Read the model definition and answer for the solid it produces. Units are mm, in the model's axes. A direction names the side the tool comes from. Coordinates: 2 decimals unless noted, no trailing zeros. Use CSV: the item, a comma, the result in double quotes.
Autodesk Inventor part; units mm, degrees
ref_plane "YZ Plane" through (0, 0, 0) normal (1, 0, 0) x (0, 1, 0)
ref_plane "XZ Plane" through (0, 0, 0) normal (0, 1, 0) x (-1, 0, 0)
ref_plane "XY Plane" through (0, 0, 0) normal (0, 0, 1) x (1, 0, 0)
sketch "Sketch1" plane through (0, 0, 0) normal (0, 0, 1) x (1, 0, 0)
  line L0 (-25, 25) -> (25, 25)
  line L1 (25, 25) -> (25, -25)
  line L2 (25, -25) -> (-25, -25)
  line L3 (-25, -25) -> (-25, 25)
  point P0 (0, 0)
  dimension "d0" = 50
  dimension "d1" = 50
  dimension "d2" = 25
  dimension "d3" = 25
extrude "Extrusion1" add sketch "Sketch1" along normal blind 5
fillet "Fillet1" radius 5 4 edges at (-25, -25, 2.5) (25, -25, 2.5) (25, 25, 2.5) (-25, 25, 2.5)
chamfer "Chamfer1" distance 2 angle 45 8 edges at (0, -25, 5) (23.5355, -23.5355, 5) (25, 0, 5) (23.5355, 23.5355, 5) (0, 25, 5) (-23.5355, 23.5355, 5) (-25, 0, 5) (-23.5355, -23.5355, 5)
sketch "Sketch3" plane through (0, 0, 0) normal (0, 0, -1) x (-1, 0, 0)
  circle A0 centre (-15, 0) radius 2.5
  circle A1 centre (15, 0) radius 2.5
  line L0 (-25, -20) -> (-25, 20)
  line L1 (25, 20) -> (25, -20)
  line L2 (20, -25) -> (-20, -25)
  point P0 (0, 0)
  point P1 (0, 0)
  dimension "d13" = 5
  dimension "d19" = 10
  dimension "d20" = 10
  dimension "d21" = 25
  dimension "d22" = 25
  dimension "d23" = 5
extrude "Extrusion3" add sketch "Sketch3" along normal blind 3
sketch "Sketch4" plane through (0, 0, 5) normal (0, 0, 1) x (1, 0, 0)
  circle A0 centre (0, 0) radius 15
  circle A1 centre (0, 0) radius 17
  dimension "d24" = 30
  dimension "d25" = 2
extrude "Extrusion4" cut sketch "Sketch4" against normal blind 1
chamfer "Chamfer3" distance 1 angle 45 2 edges at (-15, 0, 4) (-17, 0, 4)
properties part number "Top"
1. Each of these flat-tipped pins is pushed along its axis until it touches: pin 1 Ø10 at (x, y) = (-13, -8) entering from -Z; pin 2 Ø3 at (x, z) = (14, 4) entering from +Y. Where does it stop, or does it pass through?
Solutions:
pin 1,"stops at z = 0"
pin 2,"stops at y = 25"
2. A tool of negligible diameter and unlimited length cuts with its end or side. For faces 1 (the flat face through (-15, 0, -3)), 2 (the cylindrical face through (-12.5, -0.1, -1.5)), from which of +Z, -Z, +X, -X, +Y, -Y can it reach the whole face along a straight path? Write none if from no direction.
Solutions:
face 1,"-Z, +X, -X, +Y, -Y"
face 2,"-Z"
3. Find the intervals of material crossed by line 1 along Z through (x, y) = (3, -11); line 2 along Y through (x, z) = (23.5, 0.25); line 3 along Y through (x, z) = (1, 3.75), in increasing order.
Solutions:
line 1,"z = 0 to 5"
line 2,"y = -23.57 to 23.57"
line 3,"y = -24.25 to 24.25"
